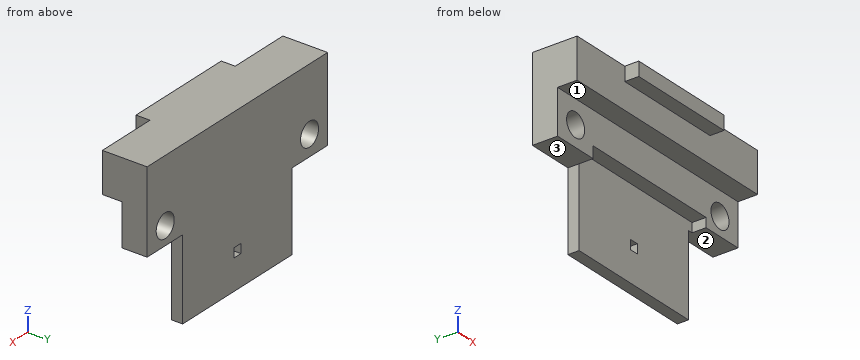
Autodesk Fusion 360 part; units mm, degrees
sketch "board contact" plane through (0, 0, 0) normal (0, 1, 0) x (1, 0, 0)
  line L0 (12.7, -1.75) -> (-12.7, -1.75)
  line L1 (-12.7, -1.75) -> (-12.7, 1.75)
  line L2 (-12.7, 1.75) -> (12.7, 1.75)
  line L3 (12.7, 1.75) -> (12.7, -1.75)
  line L4 (61.7395, 0) -> (-97.655, 0) construction
  line L5 (0, -60.5274) -> (0, 48.7233) construction
  line L6 (8.2, 2.75) -> (12.7, 2.75)
  line L7 (12.7, 2.75) -> (12.7, 1.75)
  line L8 (12.7, 1.75) -> (8.2, 1.75)
  line L9 (8.2, 1.75) -> (8.2, 2.75)
  line L10 (-12.7, 3) -> (2.45, 3)
  line L11 (2.45, 3) -> (2.45, 1.75)
  line L12 (2.45, 1.75) -> (-12.7, 1.75)
  line L13 (-12.7, 1.75) -> (-12.7, 3)
  circle A0 centre (10.16, 0.79) radius 1.27
  circle A1 centre (-10.16, 0.79) radius 1.27
  line L14 (-10.16, 0.79) -> (10.16, 0.79) construction
  line L15 (2.45, 9.25) -> (-1.95, 9.25)
  line L16 (-1.95, 9.25) -> (-1.95, 3)
  line L17 (-1.95, 3) -> (2.45, 3)
  line L18 (2.45, 3) -> (2.45, 9.25)
  line L19 (0.5, 7.19) -> (-0.5, 7.19)
  line L20 (-0.5, 7.19) -> (-0.5, 8.19)
  line L21 (-0.5, 8.19) -> (0.5, 8.19)
  line L22 (0.5, 8.19) -> (0.5, 7.19)
  line L23 (7.7, 11.45) -> (-7.7, 11.45)
  line L24 (-7.7, 11.45) -> (-7.7, -1.75)
  line L25 (-7.7, -1.75) -> (7.7, -1.75)
  line L26 (7.7, -1.75) -> (7.7, 11.45)
  line L27 (8.2, 2.75) -> (7.7, 2.75)
  line L28 (-0.5, 7.69) -> (0.5, 7.69) construction
  dimension "d1" = 3.5
  dimension "d2" = 25.4
  dimension "d3" = 4.5
  dimension "d4" = 4.5
  dimension "d7" = 4.75
  dimension "d10" = 20.32
  dimension "d11" = 2.54
  dimension "d12" = 2.54
  dimension "d13" = 10.25
  dimension "d14" = 10.75
  dimension "d15" = 11
  dimension "d17" = 1
  dimension "d18" = 1
  dimension "d20" = 5
  dimension "d21" = 5
  dimension "d22" = 13.2
  dimension "d39" = 9.44
extrude "Extrude1" add sketch "board contact" along normal blind 3.2 contours L0 L2 L3 L8 A0 L26 | L0 L2 L12 L24 L25 L26 | L2 L6 L7 L8 L9 A0 | L0 L1 L2 L12 A1 L24 | L2 L9 L26 L27 | L2 L10 L11 L15 L16 L18 L23 L24 L26 | L2 L10 L11 L12 L17 L24 | L2 L10 L12 L13 A1 L24 | L10 L15 L16 L17 L18
extrude "Extrude2" cut sketch "board contact" along normal blind 2 contours L2 L9 L26 L27 | L2 L10 L11 L15 L16 L18 L23 L24 L26 | L2 L10 L11 L12 L17 L24 | L10 L15 L16 L17 L18
sketch "vertical extension" plane through (0, 0, 0) normal (0, -1, 0) x (1, 0, 0)
  line L0 (-12.7, -3) -> (-7.7, -3)
  line L1 (-7.7, -1.75) -> (8.2, -1.75)
  line L2 (8.2, -1.75) -> (8.2, -2.75)
  line L3 (8.2, -2.75) -> (12.7, -2.75)
  line L4 (12.7, -2.75) -> (12.7, 1.75)
  line L5 (12.7, 1.75) -> (-12.7, 1.75)
  line L6 (-12.7, 1.75) -> (-12.7, -3)
  circle A0 centre (10.16, -0.79) radius 1.27
  circle A1 centre (-10.16, -0.79) radius 1.27
  line L7 (-6, 6.05) -> (6, 6.05)
  line L8 (6, 6.05) -> (6, 4.55)
  line L9 (6, 4.55) -> (-6, 4.55)
  line L10 (-6, 4.55) -> (-6, 6.05)
  line L11 (0, 1.75) -> (0, -6.45) construction
  line L12 (-12.7, 6.05) -> (12.7, 6.05)
  line L13 (12.7, 6.05) -> (12.7, 1.75)
  line L14 (12.7, 1.75) -> (-12.7, 1.75)
  line L15 (-12.7, 1.75) -> (-12.7, 6.05)
  line L16 (-7.7, -3) -> (-7.7, -1.75)
  dimension "d25" = 12
  dimension "d26" = 1.5
  dimension "d29" = 4.3
extrude "Extrude4" add sketch "vertical extension" along normal blind -3.2 and the other way blind -1.6 contours L5 L8 L9 L10 L12 L13 L14 L15 | L7 L8 L9 L10 L12
extrude "Extrude3" add sketch "vertical extension" along normal blind 3.1 contours L7 L8 L9 L10 L12
extrude "Extrude6" cut 1 faces at (-2.5667, 0, -0.6331) along direction (0, 1, 0) blind 0.5
Check sheet for the modelled part. Datum: model origin and axes. Units: mm. Face numbers are marked on the shaded views. A direction names the side the tool comes from. Round coordinates to 2 decimals unless told otherwise and drop trailing zeros. Order: outer loops, then holes, each group sorted by start corner. A loop starts at its lowest first (then second) coordinate and runs counter-clockwise, first axis right, second up.
1) Tool access check on the marked faces 1, 2 and 3. Record the directions out of +Z, -Z, +X, -X, +Y, -Y that give a thin tool (end or side, any length) a straight path to the whole face; none if there is none.
2) Section check B-B (y = 2.75). Record the boundary of the cut face in (x, z).
3) Scan lines: line 1 (X direction, y = 2.6, z = -0.79); line 2 (Z direction, x = 10.16, y = 1.6); line 3 (Z direction, x = -10.16, y = 2.1). Record each from-to range of solid material in increasing order.
4) Go/stop test with flat-tipped pins: pin 1 Ø0.8 at (y, z) = (-2.5, 5.5) entering from +X; pin 2 Ø1.6 at (x, y) = (-3.5, 1) entering from -Z; pin 3 Ø2 at (x, y) = (-11, 1.5) entering from -Z. Record where each tip stops, or that it passes through.
5) Section check D-D (z = 5.25). Record the boundary of the cut face in (x, y), and give its area (3 significant figures).
6) Section check A-A (x = 10.16). Record the boundary of the cut face in (y, z).
7) Section check C-C (x = -7.25). Record the boundary of the cut face in (y, z), and give its area (3 significant figures).
Result:
1. face 1: -Z, +X, -X, -Y
1. face 2: -Z, +X, +Y, -Y
1. face 3: -Z, -X, +Y, -Y
2. outline: (-12.7, -3) - (-7.7, -3) - (-7.7, -11.45) - (7.7, -11.45) - (7.7, -2.75) - (12.7, -2.75) - (12.7, 6.05) - (-12.7, 6.05) - close; hole circle Ø2.54 at (-10.16, -0.79); hole (-0.5, -8.19) - (0.5, -8.19) - (0.5, -7.19) - (-0.5, -7.19) - close; hole circle Ø2.54 at (10.16, -0.79)
3. line 1: x = -12.7 to -11.43, -8.89 to 8.89, 11.43 to 12.7
3. line 2: z = -2.75 to -2.06, 0.48 to 6.05
3. line 3: z = -3 to -2.06, 0.48 to 6.05
4. pin 1: stops at x = 6
4. pin 2: stops at z = -1.75
4. pin 3: stops at z = -3
5. outline: (-12.7, -1.6) - (-6, -1.6) - (-6, -3.1) - (6, -3.1) - (6, -1.6) - (12.7, -1.6) - (12.7, 3.2) - (-12.7, 3.2) - close
5. area: 140 mm2
6. outline: (-1.6, 1.75) - (0.5, 1.75) - (0.5, 0.48) - (3.2, 0.48) - (3.2, 6.05) - (-1.6, 6.05) - close; (0.5, -2.75) - (3.2, -2.75) - (3.2, -2.06) - (0.5, -2.06) - close
7. outline: (-1.6, 1.75) - (0.5, 1.75) - (0.5, -1.75) - (2, -1.75) - (2, -11.45) - (3.2, -11.45) - (3.2, 6.05) - (-1.6, 6.05) - close
7. area: 41.7 mm2
